```python
from build123d import *

# Parameters (mm, degrees)
F1_DEPTH = 50
F2_T     = -2.54


with BuildPart() as f1:
    # F0 (on Top) → F1 (new body)
    with BuildSketch(Plane.XY):
        Polygon((400, 0), (0, 0), (0, -50), (450, -50), align=None)
        Polygon((0, -50), (0, 0), (-400, 0), (-450, -50), align=None)
    extrude(amount=F1_DEPTH)

    # F2
    f2_openings = [f1.faces().sort_by_distance(p)[0] for p in [
        (425, -25, 25),
        (-425, -25, 25),
    ]]
    offset(amount=F2_T, openings=f2_openings)


solid = f1.part
```
Input: part model. Units: mm. Frame: model coordinates. A direction names the side the tool comes from. Give positions to 0.01 mm unless a question says otherwise; leave off trailing zeros. Order: outer loops, then holes, each group sorted by start corner. A loop starts at its lowest first (then second) coordinate and runs counter-clockwise, first axis right, second up.
1. Section B-B on x = -93.5. Return the cut outline in (y, z).
Derived:
outline: (-50, 0) - (0, 0) - (0, 50) - (-50, 50) - close; hole (-47.46, 2.54) - (-2.54, 2.54) - (-2.54, 47.46) - (-47.46, 47.46) - close
2. Section A-A on y = -39. Return the cut outline in (x, z).
Derived:
outline: (-439, 0) - (439, 0) - (439, 2.54) - (-439, 2.54) - close; (-439, 47.46) - (439, 47.46) - (439, 50) - (-439, 50) - close
3. Pin query (flat end, axial travel): pin 1 (2 mm diameter, centred on y = -39, z = 45, fed in from +X); pin 2 (8 mm diameter, centred on y = -44.5, z = 30.5, fed in from +X). Return the tip coordinate at first contact, or that it passes through.
Derived:
pin 1: passes through
pin 2: stops at x = 448.5
4. Mould query, pull axis Y, two halves, no side actions, for faces 3 (the flat face through (6, 0, 25)), 4 (the flat face through (-6, -25, 0)), 5 (the flat face through (-6, -25, 2.54)), 6 (the flat face through (6, -2.54, 25)). Classes: released by +Y, released by -Y, zero draft, split by the parting line, or undercut.
Derived:
face 3: released by +Y
face 4: zero draft
face 5: undercut
face 6: undercut
5. Section C-C on z = 30. Return the cut outline in (x, y).
Derived:
outline: (-450, -50) - (450, -50) - (447.46, -47.46) - (-447.46, -47.46) - close; (-402.54, -2.54) - (402.54, -2.54) - (400, 0) - (-400, 0) - close
6. Reachability of faces 1 (the flat face through (-6, -25, 47.46)), 2 (the flat face through (-6, -50, 25)) from +Z, -Z, +X, -X, +Y, -Y: full face, straight path, thin tool, end or side. Return the list, or none.
Derived:
face 1: +X, -X
face 2: +Z, -Z, +X, -X, -Y
7. Material intervals for L1, parallel to Z at x = 314.5, y = -11; L2, parallel to Y at x = -370.5, z = 24; L3, parallel to X at y = -47.5, z = 6, sorted ascending.
Derived:
L1: z = 0 to 2.54, 47.46 to 50
L2: y = -50 to -47.46, -2.54 to 0
L3: x = -447.5 to 447.5
